Design review of the part built by this model. Coordinates are the model's own, in mm. Face numbers are marked on the shaded views. A direction names the side the tool comes from. Give positions to 0.01 mm unless a question says otherwise; leave off trailing zeros. Write each loop counter-clockwise with the first axis right and the second up, starting at its lowest first coordinate (ties: lowest second). Pieces come first, ordered by that corner, then holes. Notation, with made-up numbers: (-3, 58) - (5, 58) arc R25 cw to (5, 82) - close; hole circle Ø7 at (25, 62). An arc over 180 degrees is marked (long way). Write each question's results on one line, items separated by ' | '. Start each with the question number.
from build123d import *

# Parameters (mm, degrees)
SKETCH1_R           = 10
EXTRUDE_3_8_DEPTH   = 10
CUT_EXTRUDE2_DEPTH  = 10
BOSS_EXTRUDE2_DEPTH = 10
SKETCH5_R           = 2.2
M5_DRILL_DEPTH      = 8
SKETCH7_R           = 2.2
M4_THROUGH2_DEPTH   = 10


with BuildPart() as part:
    # Sketch1 → 3/8 (new body)
    with BuildSketch(Plane.XY):
        with BuildLine():
            Line((17, 0), (17, -34.388204953))
            Line((17, -34.388204953), (-30.607305145, -34.388204953))
            Line((-30.607305145, -34.388204953), (-15.974774553, 5.814342437))
            ThreePointArc((-15.974774553, 5.814342437), (2.95201902, 16.741731801), (17, 0))
        make_face()
        Circle(SKETCH1_R, mode=Mode.SUBTRACT)
    extrude(amount=EXTRUDE_3_8_DEPTH)

    # Sketch4 → Cut-Extrude2 (cut)
    with BuildSketch(Plane.XY.offset(10)):
        with BuildLine():
            ThreePointArc((-9.762664623, -16.30001164), (-1.360957212, -18.951195093), (7.333365278, -17.527742402))
            ThreePointArc((7.333365278, -17.527742402), (11.258803332, -19.137380895), (9.649164839, -23.06281895))
            ThreePointArc((9.649164839, -23.06281895), (-1.790733174, -24.935783018), (-12.845611346, -21.447383737))
            ThreePointArc((-12.845611346, -21.447383737), (-13.877824033, -17.332224327), (-9.762664623, -16.30001164))
        make_face()
    extrude(amount=-CUT_EXTRUDE2_DEPTH, mode=Mode.SUBTRACT)

    # Sketch6 → Boss-Extrude2 (add)
    with BuildSketch(Plane.XY.offset(10)):
        Polygon((-30.607305145, -34.388204953), (-38.607305145, -34.388204953), (-38.607305145, -28.188204953), (-28.350689692, -28.188204953), align=None)
    extrude(amount=-BOSS_EXTRUDE2_DEPTH)

    # Sketch5 → M5_DRILL (cut)
    with BuildSketch(Plane.XZ.offset(34.388204953)):
        with Locations((-33.607305145, 5)):
            Circle(SKETCH5_R)
        with Locations((-8.607305145, 5)):
            Circle(SKETCH5_R)
    extrude(amount=-M5_DRILL_DEPTH, mode=Mode.SUBTRACT)

    # Sketch7 → M4_through2 (cut)
    with BuildSketch(Plane.XY.offset(10)):
        with Locations((-22.607305145, -31.288204953)):
            Circle(SKETCH7_R)
        with Locations((2.392694855, -31.288204953)):
            Circle(SKETCH7_R)
    extrude(amount=-M4_THROUGH2_DEPTH, mode=Mode.SUBTRACT)


solid = part.part
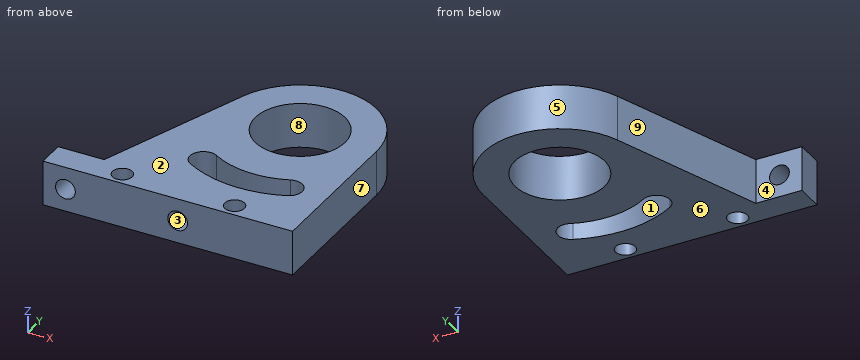
Q1. Machinability: for the marked faces 1, 2, 3, 4 and 5, which of the approach directions +Z, -Z, +X, -X, +Y, -Y give a long, thin tool a straight path to every point of the face, cutting with its end or side? Answer none if there is none.
Q2. Add section A-A on z = 5. State the section outline as (x, y) points.
Q3. Insertion check: P1, Ø3.5, axis at x = -9, z = 5, coming from the -Y side; P2, Ø1, axis at y = 1.5, z = 2, coming from the +X side; P3, Ø5, axis at x = -35, z = 5, coming from the +Y side. Each pin has a flat end and moves straight along its axis. Give the tip position at first contact, or say it passes through.
Q4. Add section B-B on y = 7.5. State the section outline as (x, z) points.
Q5. For line 1 along X through (y, z) = (-20.5, 2); line 2 along Y through (x, z) = (-13, 3.75); line 3 along Y through (x, z) = (7, 9), list the stretches that pass through material, from the lowest coordinate up. Write a range as [from, to].
Q6. The part is to be moulded in two halves that separate along X. For the marked faces 6, 7, 8 and 9, say which applies: +X half, -X half, draft (parallel to the pull), parting line (faces both ways), or undercut.
Q7. Add section D-D on z = 8.25. State the section outline as (x, y) points, plus the area to 3 significant figures.
Q8. Add section C-C on x = -4. State the section outline as (y, z) points, plus the area to 3 significant figures.
Result:
1) face 1: +Z, -Z | face 2: +Z, +X, -X, +Y, -Y | face 3: -Y | face 4: +Z, -Z, -X, +Y | face 5: +Z, -Z, +Y
2) outline: (-38.61, -34.39) - (-35.81, -34.39) - (-35.81, -28.19) - (-38.61, -28.19) - close; (-31.41, -34.39) - (-10.81, -34.39) - (-10.81, -26.39) - (-6.41, -26.39) - (-6.41, -34.39) - (17, -34.39) - (17, 0) arc R17 ccw to (-15.97, 5.81) - (-28.35, -28.19) - (-31.41, -28.19) - close; hole circle Ø4.4 at (-22.61, -31.29); hole (-12.85, -21.45) arc R25 ccw to (9.65, -23.06) arc R3 ccw to (7.33, -17.53) arc R19 cw to (-9.76, -16.3) arc R3 ccw to start; hole circle Ø20 at (0, 0); hole circle Ø4.4 at (2.39, -31.29)
3) P1: stops at y = -26.39 | P2: stops at x = 16.97 | P3: stops at y = -28.19
4) outline: (-15.26, 0) - (-6.61, 0) - (-6.61, 10) - (-15.26, 10) - close; (6.61, 0) - (15.26, 0) - (15.26, 10) - (6.61, 10) - close
5) line 1: x = [-25.55, -13.83], [11.48, 17] | line 2: y = [-34.39, -21.35], [-16.4, 10.95] | line 3: y = [-34.39, -24], [-17.66, -7.14], [7.14, 15.49]
6) face 6: draft | face 7: +X half | face 8: undercut | face 9: -X half
7) outline: (-38.61, -34.39) - (17, -34.39) - (17, 0) arc R17 ccw to (-15.97, 5.81) - (-28.35, -28.19) - (-38.61, -28.19) - close; hole circle Ø4.4 at (-22.61, -31.29); hole (-12.85, -21.45) arc R25 ccw to (9.65, -23.06) arc R3 ccw to (7.33, -17.53) arc R19 cw to (-9.76, -16.3) arc R3 ccw to start; hole circle Ø20 at (0, 0); hole circle Ø4.4 at (2.39, -31.29) | area: 1,440 mm²
8) outline: (-34.39, 0) - (-24.68, 0) - (-24.68, 10) - (-34.39, 10) - close; (-18.57, 0) - (-9.17, 0) - (-9.17, 10) - (-18.57, 10) - close; (9.17, 0) - (16.52, 0) - (16.52, 10) - (9.17, 10) - close | area: 265 mm²
